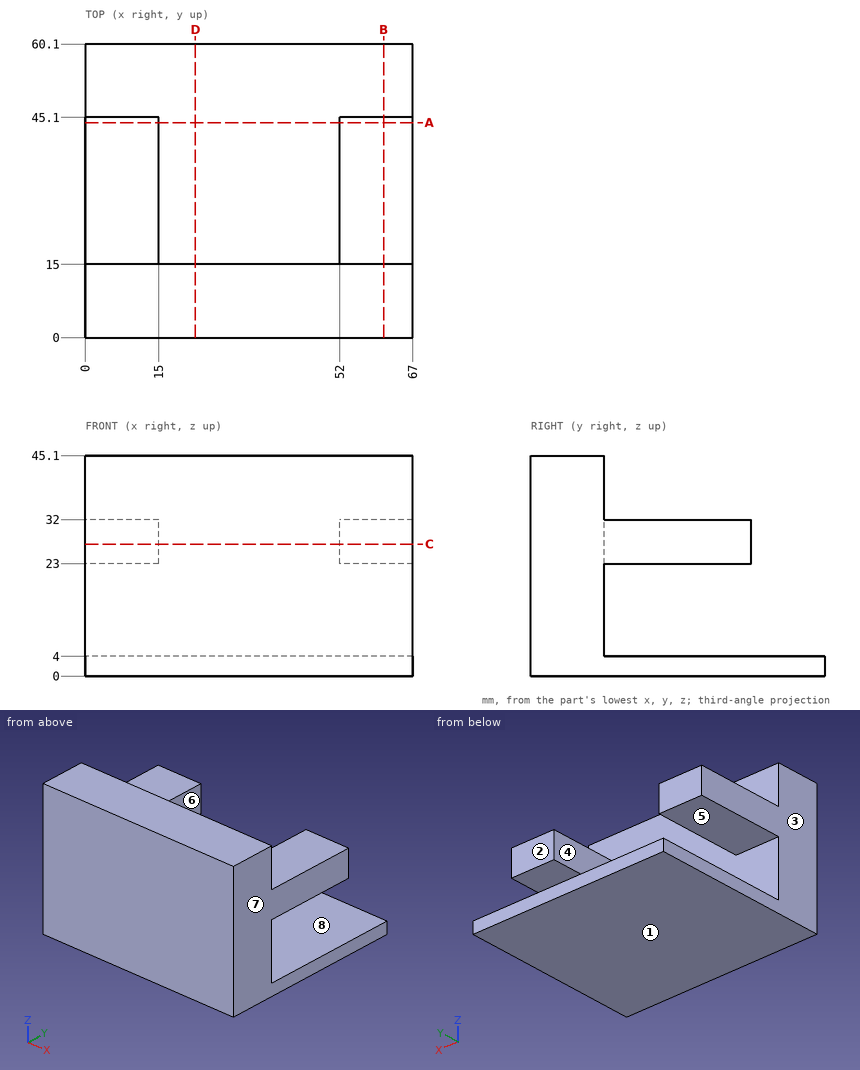
For this review, use the dimensioned drawing (mm, ordinates from the lowest corner) and the shaded views. A direction names the side the tool comes from. Round coordinates to 2 decimals unless told otherwise and drop trailing zeros. Write each loop counter-clockwise with the first axis right and the second up, starting at its lowest first coordinate (ties: lowest second). Pieces come first, ordered by that corner, then holes. Notation, with made-up numbers: (39, -22) -> (44, -22) arc R14 ccw to (44, 2) -> close; hole circle Ø4 at (-8.75, 73). An arc over 180 degrees is marked (long way). One line per item, written item: value. Start each with the question number.
Q1. Tool access review of the marked faces 1, 2, 3, 4 and 5: name each direction out of +Z, -Z, +X, -X, +Y, -Y from which nothing blocks a thin tool from reaching the whole face with its end or side.
Q2. Insertion check: P1, Ø12, axis at x = 61, y = 33.5, coming from the +Z side; P2, Ø13.5, axis at x = 30.5, y = 48, coming from the +Z side; P3, Ø4.5, axis at x = 6, z = 27, coming from the +Y side; P4, Ø2, axis at y = 38.5, z = 6.5, coming from the -X side. Each pin has a flat end and moves straight along its axis. Give the tip position at first contact, or say it passes through.
Q3. Add section D-D (x = 22.5). Give the boundary of the cut face in (y, z), then the cut area to 3 significant figures.
Q4. The part is to be moulded in two halves that separate along X. For the marked faces 6, 7 and 8, say which applies: pulls with the +X half, pulls with the -X half, needs draft (parallel to the pull), parting line crosses it, or undercut.
Q5. Add section A-A (y = 44). Give the boundary of the cut face in (x, z).
Q6. Add section C-C (z = 27). Give the boundary of the cut face in (x, y), then the cut area to 3 significant figures.
Q7. To check wall thickness, follow probe 1 along Z at (x, y) = (53.5, 22); probe 2 along X at (y, z) = (22, 23.5); probe 3 along Y at (x, z) = (56.5, 19). State the ranges of each line that lie inside material, in increasing order.
Q8. Add section B-B (x = 61). Give the boundary of the cut face in (y, z).
Response:
1. face 1: -Z, +X, -X, +Y, -Y
1. face 2: +Z, +X, -X, +Y
1. face 3: +Z, -Z, -X, +Y, -Y
1. face 4: +Z, +Y
1. face 5: +X, -X, +Y
2. P1: stops at z = 32
2. P2: stops at z = 4
2. P3: stops at y = 45.1
2. P4: passes through
3. outline: (0, 0) -> (60.1, 0) -> (60.1, 4) -> (15, 4) -> (15, 45.1) -> (0, 45.1) -> close
3. area: 857 mm^2
4. face 6: undercut
4. face 7: pulls with the +X half
4. face 8: needs draft
5. outline: (0, 0) -> (67, 0) -> (67, 4) -> (0, 4) -> close; (0, 23) -> (15, 23) -> (15, 32) -> (0, 32) -> close; (52, 23) -> (67, 23) -> (67, 32) -> (52, 32) -> close
6. outline: (0, 0) -> (67, 0) -> (67, 45.1) -> (52, 45.1) -> (52, 15) -> (15, 15) -> (15, 45.1) -> (0, 45.1) -> close
6. area: 1,910 mm^2
7. probe 1: z = 0 to 4, 23 to 32
7. probe 2: x = 0 to 15, 52 to 67
7. probe 3: y = 0 to 15
8. outline: (0, 0) -> (60.1, 0) -> (60.1, 4) -> (15, 4) -> (15, 23) -> (45.1, 23) -> (45.1, 32) -> (15, 32) -> (15, 45.1) -> (0, 45.1) -> close
